Build history of the part. All positions in model axes, mm. Give positions to 0.01 mm unless a question says otherwise; leave off trailing zeros. Loops run counter-clockwise (first coordinate to the right, second up) from the corner with the lowest first, then second, coordinate; pieces in that order, holes last. Notation, with made-up numbers: M 52.5,24.25 L 90.5,24.25 A30 ccw 90.5,61.25 Z; hole C 8.5,-5.75 d1. An arc over 180 degrees is marked long. Put each result on its own line as item: value.
```python
from build123d import *

# Parameters (mm, degrees)
F2_DEPTH = 12.7


with BuildPart() as f2:
    # F1 (on face) → F2 (new body)
    with BuildSketch(Plane.XZ):
        with BuildLine():
            Line((170.693952, 27.128556), (24.933873, 75.357101))
            ThreePointArc((24.933873, 75.357101), (-79.375, 0), (24.933873, -75.357101))
            Line((24.933873, -75.357101), (170.693952, -27.128556))
            ThreePointArc((170.693952, -27.128556), (190.292758, 0), (170.693952, 27.128556))
        make_face()
        with BuildLine():
            ThreePointArc((23.936518, -72.342817), (-76.2, 0), (23.936518, 72.342817))
            Line((23.936518, 72.342817), (169.696597, 24.114272))
            ThreePointArc((169.696597, 24.114272), (187.117758, 0), (169.696597, -24.114272))
            Line((169.696597, -24.114272), (23.936518, -72.342817))
        make_face(mode=Mode.SUBTRACT)
    extrude(amount=F2_DEPTH)


solid = f2.part
```
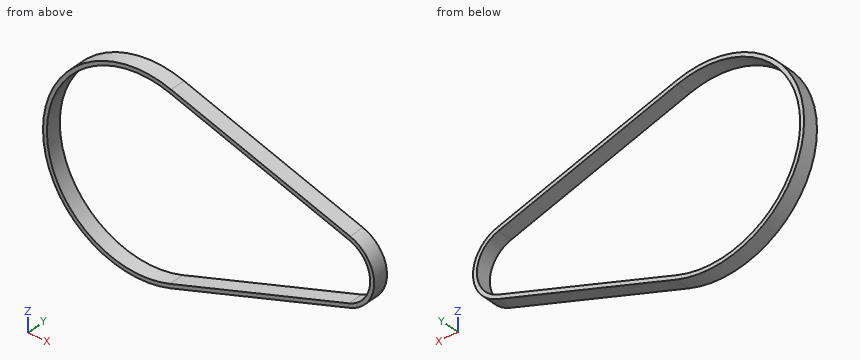
Q1. Slice it at A-A (x = 0). List the corners of the cut face in (y, z) (3 decimals).
Here are the results:
outline: M -12.7,-79.375 L 0,-79.375 L 0,-76.2 L -12.7,-76.2 Z; M -12.7,76.2 L 0,76.2 L 0,79.375 L -12.7,79.375 Z
Q2. Probe line 1 (Z direction, x = 0, y = -6.25) (3 decimals); line 2 (X direction, y = -0.5, z = 22.5); line 3 (Z direction, x = 33, y = -6.25). List the from-to ranges inside material, lowest first. Write a range as from..to.
Here are the results:
line 1: -79.375..-76.2, 76.2..79.375
line 2: -76.12..-72.8, 173.5..179.33
line 3: -72.69..-69.34, 69.34..72.69
Q3. Drop flat-ended pins along their axis: pin 1 Ø1.5 at (y, z) = (-10.5, -6) entering from -X; pin 2 Ø3 at (y, z) = (-10.5, -58) entering from -X; pin 3 Ø1 at (y, z) = (-5, -24.5) entering from -X. Give the stop position or say it passes through.
Here are the results:
pin 1: x = -79.2
pin 2: x = -55.75
pin 3: x = -75.66
Q4. Slice it at C-C (y = -3.5). List the corners of the cut face in (x, z) (3 decimals), and give its area (3 significant figures).
Here are the results:
outline: M 24.934,-75.357 L 170.694,-27.129 A28.575 ccw 170.694,27.129 L 24.934,75.357 A79.375 ccw long Z; hole M 23.937,-72.343 L 169.697,-24.114 A25.4 ccw 169.697,24.114 L 23.937,72.343 A76.2 ccw long Z
area: 2,120 mm²
Q5. Slice it at B-B (z = 0). List the corners of the cut face in (x, y) (3 decimals).
Here are the results:
outline: M -79.375,-12.7 L -76.2,-12.7 L -76.2,0 L -79.375,0 Z; M 187.118,-12.7 L 190.293,-12.7 L 190.293,0 L 187.118,0 Z
